Input: part model. Units: mm. Frame: model coordinates. A direction names the side the tool comes from. Coordinates: 2 decimals unless noted, no trailing zeros. Loops run counter-clockwise (first coordinate to the right, second up) from the corner with the lowest first, then second, coordinate; pieces in that order, holes last. Notation, with made-up numbers: (33.25, -13.75) - (65.25, -13.75) arc R17 cw to (65.25, -9.75) - close; hole circle Ø6 at (63, 88). An arc over 180 degrees is marked (long way). Use one line per item in the form item = value.
from build123d import *

# Parameters (mm, degrees)
SKETCH_1_W          = 15
SKETCH_1_H          = 15
SKETCH_1_W_2        = 13
SKETCH_1_H_2        = 13
EXTRUDE_1_DEPTH     = 292.5
SKETCH_2_R          = 1.6
CUT_EXTRUDE_1_DEPTH = 293.980374769
SKETCH_3_R          = 1.6
CUT_EXTRUDE_2_DEPTH = 293.980374769


with BuildPart() as part:
    # 草图1 → 拉伸-薄壁1 (new body)
    with BuildSketch(Plane(origin=(0, 0, 0), x_dir=(1, 0, 0), z_dir=(0, 1, 0))):
        Rectangle(SKETCH_1_W, SKETCH_1_H)
        Rectangle(SKETCH_1_W_2, SKETCH_1_H_2, mode=Mode.SUBTRACT)
    extrude(amount=EXTRUDE_1_DEPTH)

    # 草图2 → 切除-拉伸1 (cut, through all)
    with BuildSketch(Plane.XY.offset(7.5)):
        with Locations((0, 7.5)):
            Circle(SKETCH_2_R)
        with Locations((0, 27.5)):
            Circle(SKETCH_2_R)
        with Locations(Location((0, 265, 0), (0, 0, 180))):
            Circle(SKETCH_2_R)
        with Locations(Location((0, 285, 0), (0, 0, 180))):
            Circle(SKETCH_2_R)
    extrude(amount=-CUT_EXTRUDE_1_DEPTH, mode=Mode.SUBTRACT)

    # 草图3 → 切除-拉伸2 (cut, through all)
    with BuildSketch(Plane(origin=(7.5, 0, 0), x_dir=(0, 0, -1), z_dir=(1, 0, 0))):
        with Locations((0, 27.5)):
            Circle(SKETCH_3_R)
        with Locations((0, 47.5)):
            Circle(SKETCH_3_R)
        with Locations((0, 67.5)):
            Circle(SKETCH_3_R)
    extrude(amount=-CUT_EXTRUDE_2_DEPTH, mode=Mode.SUBTRACT)


solid = part.part
Q1. Pull-direction query (Z, two-part tool) for faces 3 (the flat face through (0, 144, -6.5)), 4 (the flat face through (-7, 292.5, 0)), 5 (the flat face through (0, 144, -7.5)); classes: pulls with the +Z half, pulls with the -Z half, needs draft (parallel to the pull), parting line crosses it, or undercut.
Check values:
face_3 = undercut
face_4 = needs draft
face_5 = pulls with the -Z half
Q2. Set-up query: faces 1 (the flat face through (-6.5, 144, 0)), 2 (the flat face through (-7, 0, 0)). Return all of +Z, -Z, +X, -X, +Y, -Y with unobstructed straight access to the full face (end or side cutting, diameter ignored); none if empty.
Check values:
face_1 = +Y, -Y
face_2 = +Z, -Z, +X, -X, -Y
Q3. Ray query, line 1 along Y through (x, z) = (0, 6.85); line 2 along X through (y, z) = (224, 5); line 3 along X through (y, z) = (285, -6.85). Return the intervals inside material, ascending. Write a range as [from, to].
Check values:
line_1 = [0, 5.9], [9.1, 25.9], [29.1, 263.4], [266.6, 283.4], [286.6, 292.5]
line_2 = [-7.5, -6.5], [6.5, 7.5]
line_3 = [-7.5, -1.6], [1.6, 7.5]
Q4. First-contact query: P1, Ø3, axis at y = 47.5, z = 0, coming from the -X side. Flat tip, straight axial feed; report the tip coordinate or a pass-through.
Check values:
P1 = through
Q5. Cut plane A-A, the plane y = 230. Return loops of the section in (x, z).
Check values:
outline = (-7.5, -7.5) - (7.5, -7.5) - (7.5, 7.5) - (-7.5, 7.5) - close; hole (-6.5, -6.5) - (6.5, -6.5) - (6.5, 6.5) - (-6.5, 6.5) - close
